from build123d import *

# Parameters (mm, degrees)
SKETCH1_R           = 2.5
BOSS_EXTRUDE1_DEPTH = 3
BOSS_EXTRUDE2_DEPTH = 8
SKETCH4_R           = 1.7
BOSS_EXTRUDE3_DEPTH = 8
CUT_EXTRUDE1_DEPTH  = 4
SKETCH7_R           = 2.5
CUT_EXTRUDE2_DEPTH  = 10


with BuildPart() as part:
    # Sketch1 → Boss-Extrude1 (new body)
    with BuildSketch(Plane(origin=(0, 0, 0), x_dir=(1, 0, 0), z_dir=(0, 1, 0))):
        with BuildLine():
            ThreePointArc((4.727449491, 10.04296875), (0, 13.15), (-4.727449491, 10.04296875))
            ThreePointArc((-4.727449491, 10.04296875), (-11.1, 0), (-4.727449491, -10.04296875))
            ThreePointArc((-4.727449491, -10.04296875), (0, -13.15), (4.727449491, -10.04296875))
            ThreePointArc((4.727449491, -10.04296875), (11.1, 0), (4.727449491, 10.04296875))
        make_face()
        with Locations(Location((0, -8, 0), (0, 0, 270))):
            Circle(SKETCH1_R, mode=Mode.SUBTRACT)
        with Locations(Location((0, 8, 0), (0, 0, 270))):
            Circle(SKETCH1_R, mode=Mode.SUBTRACT)
    extrude(amount=BOSS_EXTRUDE1_DEPTH)

    # Sketch3 → Boss-Extrude2 (add)
    with BuildSketch(Plane(origin=(0, 3, 0), x_dir=(1, 0, 0), z_dir=(0, 1, 0))):
        with BuildLine():
            ThreePointArc((4.727449491, -10.04296875), (11.1, 0), (4.727449491, 10.04296875))
            ThreePointArc((4.727449491, 10.04296875), (0, 13.15), (-4.727449491, 10.04296875))
            ThreePointArc((-4.727449491, 10.04296875), (-11.1, 0), (-4.727449491, -10.04296875))
            ThreePointArc((-4.727449491, -10.04296875), (0, -13.15), (4.727449491, -10.04296875))
        make_face()
        with BuildLine():
            ThreePointArc((3.106861323, 7.48046875), (8.1, 0), (3.106861323, -7.48046875))
            ThreePointArc((3.106861323, -7.48046875), (0, -11.15), (-3.106861323, -7.48046875))
            ThreePointArc((-3.106861323, -7.48046875), (-8.1, 0), (-3.106861323, 7.48046875))
            ThreePointArc((-3.106861323, 7.48046875), (0, 11.15), (3.106861323, 7.48046875))
        make_face(mode=Mode.SUBTRACT)
    extrude(amount=BOSS_EXTRUDE2_DEPTH)

    # Sketch4 → Boss-Extrude3 (add)
    # profile 1 of 8: a face of its own
    with BuildSketch(Plane.XZ):
        with BuildLine():
            Line((10.055844072, -4.7), (15, -4.7))
            ThreePointArc((15, -4.7), (12.597919106, -4.039802889), (10.870666667, -2.244683992))
            ThreePointArc((10.870666667, -2.244683992), (10.53503, -3.496161166), (10.055844072, -4.7))
        make_face()
    # profile 2 of 8: a face of its own
    with BuildSketch(Plane.XZ):
        with BuildLine():
            ThreePointArc((10.870666667, 2.244683992), (12.597919106, 4.039802889), (15, 4.7))
            Line((15, 4.7), (10.055844072, 4.7))
            ThreePointArc((10.055844072, 4.7), (10.53503, 3.496161166), (10.870666667, 2.244683992))
        make_face()
    # profile 3 of 8: a face of its own
    with BuildSketch(Plane.XZ):
        with BuildLine():
            ThreePointArc((10.870666667, -2.244683992), (12.597919106, -4.039802889), (15, -4.7))
            ThreePointArc((15, -4.7), (18.323401872, -3.323401872), (19.7, 0))
            ThreePointArc((19.7, 0), (18.323401872, 3.323401872), (15, 4.7))
            ThreePointArc((15, 4.7), (12.597919106, 4.039802889), (10.870666667, 2.244683992))
            ThreePointArc((10.870666667, 2.244683992), (11.1, 0), (10.870666667, -2.244683992))
        make_face()
        with Locations(Location((15, 0, 0), (0, 0, 270))):
            Circle(SKETCH4_R, mode=Mode.SUBTRACT)
    # profile 4 of 8: a face of its own
    with BuildSketch(Plane.XZ):
        with BuildLine():
            ThreePointArc((-10.870666667, 2.244683992), (-12.597919106, 4.039802889), (-15, 4.7))
            ThreePointArc((-15, 4.7), (-19.7, 0), (-15, -4.7))
            ThreePointArc((-15, -4.7), (-12.597919106, -4.039802889), (-10.870666667, -2.244683992))
            ThreePointArc((-10.870666667, -2.244683992), (-11.1, 0), (-10.870666667, 2.244683992))
        make_face()
        with Locations(Location((-15, 0, 0), (0, 0, 270))):
            Circle(SKETCH4_R, mode=Mode.SUBTRACT)
    # profile 5 of 8: a face of its own
    with BuildSketch(Plane.XZ):
        with BuildLine():
            ThreePointArc((-10.870666667, -2.244683992), (-12.597919106, -4.039802889), (-15, -4.7))
            Line((-15, -4.7), (-10.055844072, -4.7))
            ThreePointArc((-10.055844072, -4.7), (-10.53503, -3.496161166), (-10.870666667, -2.244683992))
        make_face()
    # profile 6 of 8: a face of its own
    with BuildSketch(Plane.XZ):
        with BuildLine():
            Line((-10.055844072, 4.7), (-15, 4.7))
            ThreePointArc((-15, 4.7), (-12.597919106, 4.039802889), (-10.870666667, 2.244683992))
            ThreePointArc((-10.870666667, 2.244683992), (-10.53503, 3.496161166), (-10.055844072, 4.7))
        make_face()
    # profile 7 of 8: a face of its own
    with BuildSketch(Plane.XZ):
        with BuildLine():
            ThreePointArc((-10.3, 0), (-10.444900294, 1.158044328), (-10.870666667, 2.244683992))
            ThreePointArc((-10.870666667, 2.244683992), (-11.1, 0), (-10.870666667, -2.244683992))
            ThreePointArc((-10.870666667, -2.244683992), (-10.444900294, -1.158044328), (-10.3, 0))
        make_face()
    # profile 8 of 8: a face of its own
    with BuildSketch(Plane.XZ):
        with BuildLine():
            ThreePointArc((10.870666667, 2.244683992), (10.3, 0), (10.870666667, -2.244683992))
            ThreePointArc((10.870666667, -2.244683992), (11.1, 0), (10.870666667, 2.244683992))
        make_face()
    extrude(amount=-BOSS_EXTRUDE3_DEPTH)

    # Sketch5 → Cut-Extrude1 (cut)
    with BuildSketch(Plane(origin=(0, 8, 0), x_dir=(1, 0, 0), z_dir=(0, 1, 0))):
        Polygon((-15, -3.348631561), (-12.1, -1.674315781), (-12.1, 1.674315781), (-15, 3.348631561), (-17.9, 1.674315781), (-17.9, -1.674315781), align=None)
        Polygon((15, -3.348631561), (17.9, -1.674315781), (17.9, 1.674315781), (15, 3.348631561), (12.1, 1.674315781), (12.1, -1.674315781), align=None)
    extrude(amount=-CUT_EXTRUDE1_DEPTH, mode=Mode.SUBTRACT)

    # Sketch7 → Cut-Extrude2 (cut)
    with BuildSketch(Plane(origin=(0, 3, 0), x_dir=(1, 0, 0), z_dir=(0, 1, 0))):
        with Locations((4.242640687, 4.242640687)):
            Circle(SKETCH7_R)
        with Locations((4.242640687, -4.242640687)):
            Circle(SKETCH7_R)
        with Locations((-4.242640687, -4.242640687)):
            Circle(SKETCH7_R)
        with Locations((-4.242640687, 4.242640687)):
            Circle(SKETCH7_R)
    extrude(amount=CUT_EXTRUDE2_DEPTH, mode=Mode.SUBTRACT)


solid = part.part
Geometry: final body of the model. Coordinates: model frame, mm. A direction names the side the tool comes from. Give positions to 0.01 mm unless a question says otherwise; leave off trailing zeros. Loops run counter-clockwise (first coordinate to the right, second up) from the corner with the lowest first, then second, coordinate; pieces in that order, holes last. Notation, with made-up numbers: M -3,31.25 L 2,31.25 A21 cw 2,55.25 Z; hole C -24.5,82.5 d2. An arc over 180 degrees is marked long. Put each result on its own line as item: value. Start each with the question number.
1) Cut plane A-A (x = 0). Output: boundary loops of the cut face in (y, z).
2) Pull-direction query (X, two-part tool) for faces 4 (the cylindrical face through (0.1, 1.5, -10.5)), 5 (the flat face through (12, 4, -4.7)), 6 (the cylindrical face through (-0.08, 5.42, 13.15)); classes: pulls with the +X half, pulls with the -X half, needs draft (parallel to the pull), parting line crosses it, or undercut.
3) Access query for faces 1 (the flat face through (0, 0, 0)), 2 (the flat face through (-13.53, 6.03, -2.5)), 3 (the flat face through (13, 4, 4.7)). Directions: +Z, -Z, +X, -X, +Y, -Y. A direction counts if a zero-diameter tool reaches every point of the face in a straight line with its end or side. Return the directions, or none.
4) Contact query for flat-ended pins moving along their axis: pin 1 (2.5 mm diameter, centred on x = 12.5, y = 5, fed in from +Z); pin 2 (3 mm diameter, centred on x = -14, z = 1.5, fed in from +Y); pin 3 (3 mm diameter, centred on x = -7, y = 8.5, fed in from +Z); pin 4 (4 mm diameter, centred on x = 0, z = 8, fed in from -Y). Output: stop coordinate, or through.
5) Cut plane B-B (z = 9.5). Output: boundary loops of the cut face in (x, y).
6) Cut plane D-D (z = -8). Output: boundary loops of the cut face in (x, y), then the cut area to 3 significant figures.
7) Ray query, line 1 along Z through (x, y) = (-4.5, 3.5); line 2 along X through (y, z) = (2, -1.25); line 3 along Y through (x, z) = (-1.5, -5). Return the intervals inside material, ascending.
8) Cut plane C-C (y = 2.25). Output: boundary loops of the cut face in (x, z), then the cut area to 3 significant figures.
Verdict:
1. outline: M 0,-13.15 L 11,-13.15 L 11,-11.15 L 3,-11.15 L 3,-10.5 L 0,-10.5 Z; M 0,-5.5 L 3,-5.5 L 3,5.5 L 0,5.5 Z; M 0,10.5 L 3,10.5 L 3,11.15 L 11,11.15 L 11,13.15 L 0,13.15 Z
2. face 4: undercut
2. face 5: needs draft
2. face 6: parting line crosses it
3. face 1: +Z, -Z, +X, -X, -Y
3. face 2: +Y
3. face 3: +Z, +X, +Y, -Y
4. pin 1: z = 4.7
4. pin 2: y = 8
4. pin 3: z = 9.64
4. pin 4: through
5. outline: M -5.74,0 L -2,0 L -2,3 L -2.77,3 L -2.77,11 L -5.74,11 Z; M 2,0 L 5.74,0 L 5.74,11 L 2.77,11 L 2.77,3 L 2,3 Z
6. outline: M -7.69,0 L -2.5,0 L -2.5,3 L -3.15,3 L -3.15,11 L -7.69,11 Z; M 2.5,0 L 7.69,0 L 7.69,11 L 3.15,11 L 3.15,3 L 2.5,3 Z
6. area: 104 mm2
7. line 1: -10.5 to -6.73, 6.73 to 10.5
7. line 2: -19.53 to -16.15, -13.85 to 13.85, 16.15 to 19.53
7. line 3: 0 to 3
8. outline: M -15,-4.7 L -10.06,-4.7 A11.1 ccw -4.73,-10.04 A5.15 ccw 4.73,-10.04 A11.1 ccw 10.06,-4.7 L 15,-4.7 A4.7 ccw 15,4.7 L 10.06,4.7 A11.1 ccw 4.73,10.04 A5.15 ccw -4.73,10.04 A11.1 ccw -10.06,4.7 L -15,4.7 A4.7 ccw Z; hole C -15,0 d3.4; hole C 0,-8 d5; hole C 0,8 d5; hole C 15,0 d3.4
8. area: 508 mm2
